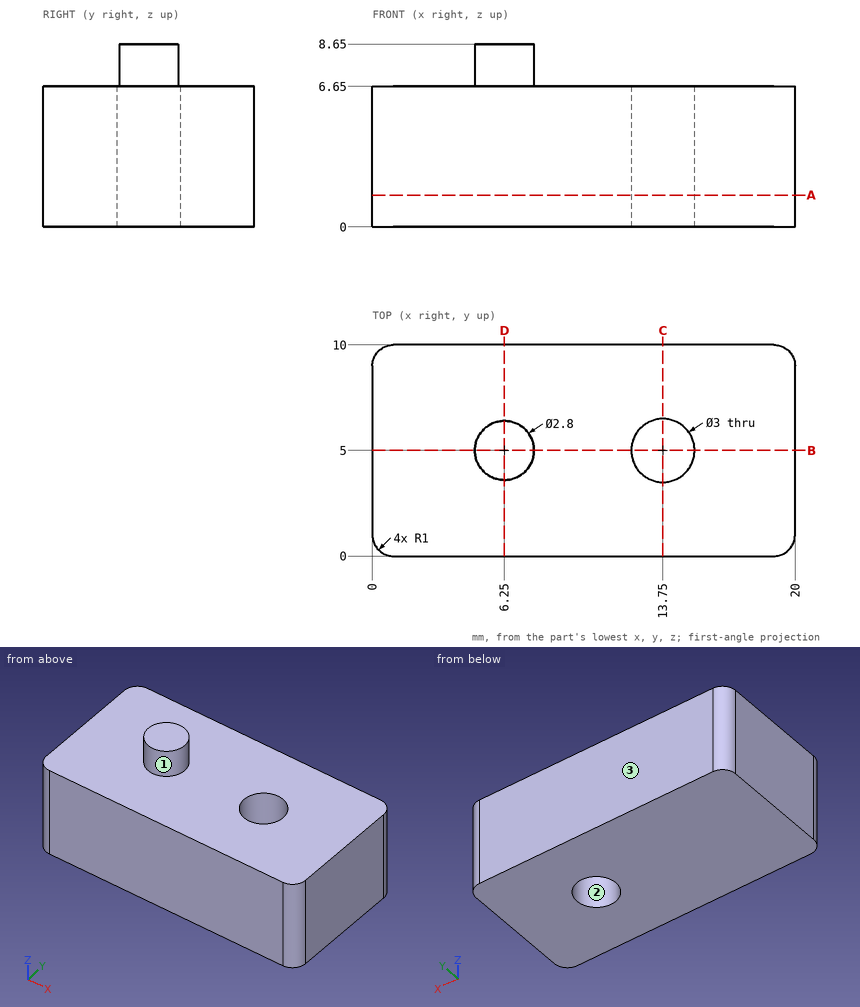
Can you work these out from the drawing? Everything is in mm from the part's minimum corner. Coordinates: 2 decimals unless noted, no trailing zeros. Loops run counter-clockwise (first coordinate to the right, second up) from the corner with the lowest first, then second, coordinate; pieces in that order, holes last.
1. Imagine slicing it at B-B, the plane y = 5. Please give me the cut outline in (x, z), and give its area (3 significant figures).
2. I need wall thicknesses on L1, parallel to Y at x = 13.75, z = 2.5; L2, parallel to Z at x = 14.5, y = 0.75; L3, parallel to X at y = 6, z = 4.75. Which ranges of each line are inside material? Lowest first, please.
3. Imagine slicing it at D-D, the plane x = 6.25. Please give me the cut outline in (y, z), and give its area (3 significant figures).
4. For P1, Ø1.5, axis at y = 6.5, z = 7.5, coming from the +X side; P2, Ø3, axis at x = 2.5, y = 1.5, coming from the +Z side; P3, Ø2, axis at y = 6.5, z = 4, coming from the -X side, each with a flat end and sliding along its axis, tell me the tip position at first contact or that it passes through.
5. Imagine slicing it at C-C, the plane x = 13.75. Please give me the cut outline in (y, z), and give its area (4 significant figures).
6. Imagine slicing it at A-A, the plane z = 1.5. Please give me the cut outline in (x, y).
7. If we mould it in two halves opening along X, with no side actions, what happens to the marked faces 1, 2 and 3? For each: pulls with the +X half, pulls with the -X half, needs draft (parallel to the pull), parting line crosses it, or undercut.
Taken from the geometry:
1. outline: (0, 0) - (12.25, 0) - (12.25, 6.65) - (7.65, 6.65) - (7.65, 8.65) - (4.85, 8.65) - (4.85, 6.65) - (0, 6.65) - close; (15.25, 0) - (20, 0) - (20, 6.65) - (15.25, 6.65) - close
1. area: 119 mm2
2. L1: y = 0 to 3.5, 6.5 to 10
2. L2: z = 0 to 6.65
2. L3: x = 0 to 12.63, 14.87 to 20
3. outline: (0, 0) - (10, 0) - (10, 6.65) - (6.4, 6.65) - (6.4, 8.65) - (3.6, 8.65) - (3.6, 6.65) - (0, 6.65) - close
3. area: 72.1 mm2
4. P1: stops at x = 7.43
4. P2: stops at z = 6.65
4. P3: stops at x = 0
5. outline: (0, 0) - (3.5, 0) - (3.5, 6.65) - (0, 6.65) - close; (6.5, 0) - (10, 0) - (10, 6.65) - (6.5, 6.65) - close
5. area: 46.55 mm2
6. outline: (0, 1) arc R1 ccw to (1, 0) - (19, 0) arc R1 ccw to (20, 1) - (20, 9) arc R1 ccw to (19, 10) - (1, 10) arc R1 ccw to (0, 9) - close; hole circle Ø3 at (13.75, 5)
7. face 1: parting line crosses it
7. face 2: undercut
7. face 3: needs draft
